from build123d import *

# Parameters (mm, degrees)
BOSS_EXTRUDE1_DEPTH         = 38
M3_5X0_6_TAPPED_HOLE2_D     = 2.9
M3_5X0_6_TAPPED_HOLE2_DEPTH = 4.5
M3_5X0_6_TAPPED_HOLE2_TIP   = 0.871247898
M8_TAPPED_HOLE1_D           = 6.8


with BuildPart() as part:
    # Sketch2 → Boss-Extrude1 (new body)
    with BuildSketch(Plane(origin=(0, 0, 0), x_dir=(1, 0, 0), z_dir=(0, 1, 0))):
        with BuildLine():
            Line((-22.139889534, 9.97315624), (10.160110466, 9.97315624))
            ThreePointArc((10.160110466, 9.97315624), (13.695644372, 8.508690146), (15.160110466, 4.97315624))
            Line((15.160110466, 4.97315624), (15.160110466, -27.32684376))
            ThreePointArc((15.160110466, -27.32684376), (13.695644372, -30.862377666), (10.160110466, -32.32684376))
            Line((10.160110466, -32.32684376), (-22.139889534, -32.32684376))
            ThreePointArc((-22.139889534, -32.32684376), (-25.67542344, -30.862377666), (-27.139889534, -27.32684376))
            Line((-27.139889534, -27.32684376), (-27.139889534, 4.97315624))
            ThreePointArc((-27.139889534, 4.97315624), (-25.67542344, 8.508690146), (-22.139889534, 9.97315624))
        make_face()
    extrude(amount=BOSS_EXTRUDE1_DEPTH)

    # M3.5x0.6 Tapped Hole2
    with Locations(Plane(origin=(-21.489889534, 38, 26.67684376), x_dir=(0, 0, 1), z_dir=(0, 1, 0))):
        with Locations((0, 0), (-31, 0), (-31, 31), (0, 31)):
            Hole(M3_5X0_6_TAPPED_HOLE2_D / 2, depth=M3_5X0_6_TAPPED_HOLE2_DEPTH)
            with Locations((0, 0, -(M3_5X0_6_TAPPED_HOLE2_DEPTH + M3_5X0_6_TAPPED_HOLE2_TIP / 2))):  # 118° drill point
                Cone(0, M3_5X0_6_TAPPED_HOLE2_D / 2, M3_5X0_6_TAPPED_HOLE2_TIP, mode=Mode.SUBTRACT)

    # M8 Tapped Hole1 (through all)
    with Locations(Plane(origin=(-6.693665392, 38, 11.655067781), x_dir=(0, 0, 1), z_dir=(0, 1, 0))):
        with Locations((0, 0)):
            Hole(M8_TAPPED_HOLE1_D / 2)


solid = part.part
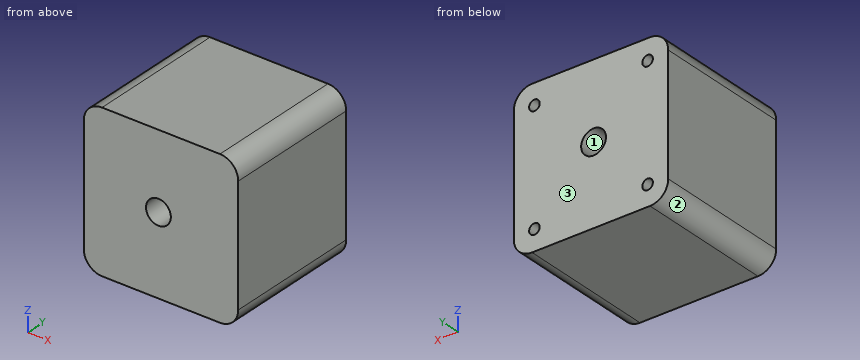
Source: CAD feature listing. Evaluate the final solid. Frame: model axes, mm. Face numbers are marked on the shaded views. Coordinates: 2 decimals unless noted, no trailing zeros. Order: outer loops, then holes, each group sorted by start corner. A loop starts at its lowest first (then second) coordinate and runs counter-clockwise, first axis right, second up. Notation, with made-up numbers: M 77.5,-8.5 L 135.5,-8.5 A22 ccw 135.5,14.5 Z; hole C -29,80 d1. An arc over 180 degrees is marked long. Write each question's results on one line, items separated by ' | '. Start each with the question number.
Item 1: Draft query along Z for the marked faces 1, 2 and 3. Return one class per face: pulls with the +Z half, pulls with the -Z half, needs draft (parallel to the pull), parting line crosses it, or undercut.
Item 2: First-contact query: pin 1 Ø2.5 at (x, z) = (9.51, 26.68) entering from +Y. Flat tip, straight axial feed; report the tip coordinate or a pass-through.
Item 3: Line query: probe 1 along X at (y, z) = (35.5, -3); probe 2 along Z at (x, y) = (-7.5, 30); probe 3 along X at (y, z) = (26, 30). Output: solid intervals per line, ascending.
Item 4: Cut plane A-A (y = 17.5). Return loops of the section in (x, z).
Checked values:
1) face 1: undercut | face 2: pulls with the -Z half | face 3: needs draft
2) pin 1: stops at y = 33.38
3) probe 1: x = -27.14 to -22.08, -20.9 to 8.92, 10.1 to 15.16 | probe 2: z = -9.97 to 8.35, 14.96 to 32.33 | probe 3: x = -26.37 to 14.39
4) outline: M -27.14,-4.97 A5 ccw -22.14,-9.97 L 10.16,-9.97 A5 ccw 15.16,-4.97 L 15.16,27.33 A5 ccw 10.16,32.33 L -22.14,32.33 A5 ccw -27.14,27.33 Z; hole C -6.69,11.66 d6.8
